from build123d import *

# Parameters (mm, degrees)
EXTRUDE_2_DEPTH     = 37.5
SKETCH_2_W          = 10
SKETCH_2_H          = 15
CUT_EXTRUDE_2_DEPTH = 20
FILLET_1_R          = 10
FILLET_2_R          = 10
CUT_EXTRUDE_3_DEPTH = 15


with BuildPart() as part:
    # 草图1 → 凸台-拉伸2 (new body, symmetric)
    with BuildSketch(Plane.XY):
        with BuildLine():
            Line((0, 0), (52.859259966, 0))
            ThreePointArc((52.859259966, 0), (56.955020188, 2.132117818), (57.55772307, 6.710100717))
            Line((57.55772307, 6.710100717), (38.189406423, 59.924113358))
            ThreePointArc((38.189406423, 59.924113358), (33.926722033, 63.194986132), (29.1608163, 60.714012641))
            Line((29.1608163, 60.714012641), (9.522083601, 26.698729811))
            Line((9.522083601, 26.698729811), (-1.736246648, 33.198729811))
            Line((-1.736246648, 33.198729811), (1.763753352, 39.260907637))
            Line((1.763753352, 39.260907637), (4.361829564, 37.760907637))
            Line((4.361829564, 37.760907637), (2.361829564, 34.296806022))
            Line((2.361829564, 34.296806022), (8.42400739, 30.796806022))
            Line((8.42400739, 30.796806022), (26.562740089, 62.214012641))
            ThreePointArc((26.562740089, 62.214012641), (34.188189261, 66.183570226), (41.008484285, 60.950173788))
            Line((41.008484285, 60.950173788), (60.376800933, 7.736161147))
            ThreePointArc((60.376800933, 7.736161147), (59.412476321, 0.411388509), (52.859259966, -3))
            Line((52.859259966, -3), (0, -3))
            Line((0, -3), (0, 0))
        make_face()
    extrude(amount=EXTRUDE_2_DEPTH, both=True)

    # 草图2 → 切除-拉伸2 (cut)
    with BuildSketch(Plane(origin=(-15.677656681, 9.051499305, 0), x_dir=(0, 0, 1), z_dir=(-0.866025404, 0.5, 0))):
        with Locations((0, 27.882820066)):
            Rectangle(SKETCH_2_W, SKETCH_2_H)
    extrude(amount=-CUT_EXTRUDE_2_DEPTH, mode=Mode.SUBTRACT)

    # 圆角1
    fillet_1_edges = [part.edges().sort_by_distance(p)[0] for p in [
        (0, -1.5, -37.5),
    ]]
    fillet(fillet_1_edges, radius=FILLET_1_R)

    # 圆角2
    fillet_2_edges = [part.edges().sort_by_distance(p)[0] for p in [
        (0, -1.5, 37.5),
    ]]
    fillet(fillet_2_edges, radius=FILLET_2_R)

    # 草图3 → 切除-拉伸3 (cut)
    with BuildSketch(Plane(origin=(-7.017402643, 4.051499305, 0), x_dir=(0, 0, 1), z_dir=(-0.866025404, 0.5, 0))):
        Polygon((-1.341883091, 59.052563915), (-10.735064726, 45.214394542), (6.122341602, 45.214394542), align=None)
    extrude(amount=-CUT_EXTRUDE_3_DEPTH, mode=Mode.SUBTRACT)


solid = part.part
Can you work these out from the model? Positions are in its coordinate system, mm. A direction names the side the tool comes from. Coordinates: 2 decimals unless noted, no trailing zeros. Write each loop counter-clockwise with the first axis right and the second up, starting at its lowest first coordinate (ties: lowest second). Pieces come first, ordered by that corner, then holes.
Q1. Imagine slicing it at A-A, the plane x = 33.5. List the corners of the cut face in (y, z) for me, plus the area to 3 significant figures.
Results found:
outline: (-3, -37.5) - (0, -37.5) - (0, 37.5) - (-3, 37.5) - close; (63.21, -37.5) - (66.21, -37.5) - (66.21, 37.5) - (63.21, 37.5) - close
area: 450 mm2
Q2. Imagine slicing it at D-D, the plane z = -8. List the corners of the cut face in (x, y) for me.
Results found:
outline: (-1.74, 33.2) - (9.52, 26.7) - (18.19, 41.71) - (15.59, 43.21) - (8.42, 30.8) - (2.36, 34.3) - (4.36, 37.76) - (1.76, 39.26) - close; (0, -3) - (52.86, -3) arc R8 ccw to (60.38, 7.74) - (41.01, 60.95) arc R8 ccw to (26.56, 62.21) - (17.6, 46.7) - (20.2, 45.2) - (29.16, 60.71) arc R5 cw to (38.19, 59.92) - (57.56, 6.71) arc R5 cw to (52.86, 0) - (0, 0) - close
Q3. Which directions (+Z, -Z, +X, -X, +Y, -Y) give clear straight access to the entire face, cutting with the end or side of a thin tool? Please do faces 4 (the face through (3.045, 38.521, -21.022)), 5 (the face through (0, -2, 0)), 6 (the face through (3.972, 29.903, -21.022)), 7 (the face through (48, 34, 37.5)), 8 (the face through (17.3, 40.17, 0.52)).
Results found:
face 4: +Z, -Z, +Y
face 5: +Z, -Z, -X, -Y
face 6: +Z, -Z, -X
face 7: +Z, +X, -X, +Y, -Y
face 8: +Z, -Z
Q4. If we mould it in two halves opening along Z, with no side actions, what happens to faces 1 (the face through (-0.01, 36.19, 21.48)), 2 (the face through (11.955, 33.954, -0.07)), 3 (the face through (2.85, -1.48, 34.49))? For each: +Z half, -Z half, draft (parallel to the pull), parting line (faces both ways), or undercut.
Results found:
face 1: draft
face 2: undercut
face 3: +Z half
Q5. Imagine slicing it at B-B, the plane z = 20.5. List the corners of the cut face in (x, y) for me.
Results found:
outline: (-1.74, 33.2) - (9.52, 26.7) - (29.16, 60.71) arc R5 cw to (38.19, 59.92) - (57.56, 6.71) arc R5 cw to (52.86, 0) - (0, 0) - (0, -3) - (52.86, -3) arc R8 ccw to (60.38, 7.74) - (41.01, 60.95) arc R8 ccw to (26.56, 62.21) - (8.42, 30.8) - (2.36, 34.3) - (4.36, 37.76) - (1.76, 39.26) - close
Q6. Imagine slicing it at C-C, the plane y = 28. List the corners of the cut face in (x, z) for me, plus the area to 3 significant figures.
Results found:
outline: (7.27, -37.5) - (10.27, -37.5) - (10.27, -5) - (7.27, -5) - close; (7.27, 5) - (10.27, 5) - (10.27, 37.5) - (7.27, 37.5) - close; (49.81, -37.5) - (53, -37.5) - (53, 37.5) - (49.81, 37.5) - close
area: 435 mm2
Q7. Please list where these lines run through material, in increasing order: L1, parallel to X at y = 33.5, z = 20; L2, parallel to Y at x = 2.5, z = -19; L3, parallel to X at y = 34.5, z = -29.
Results found:
L1: x = -1.56 to 3.74, 9.98 to 13.45, 47.81 to 51
L2: y = -3 to 0, 30.75 to 34.22, 34.54 to 38.84
L3: x = -0.98 to 2.48, 10.56 to 14.03, 47.44 to 50.64
Q8. For P1, Ø1.5, axis at y = -1.5, z = -2.5, coming from the -X side; P2, Ø4, axis at x = 30.5, z = -8, coming from the +Y side; P3, Ø8, axis at y = 37, z = -21, coming from the +X side; P4, Ø8, axis at x = 38.5, y = 6, coming from the -Z side, each with a flat end and sliding along its axis, tell me the tip position at first contact or that it passes through.
Results found:
P1: stops at x = 0
P2: stops at y = 66.15
P3: stops at x = 51.18
P4: passes through
